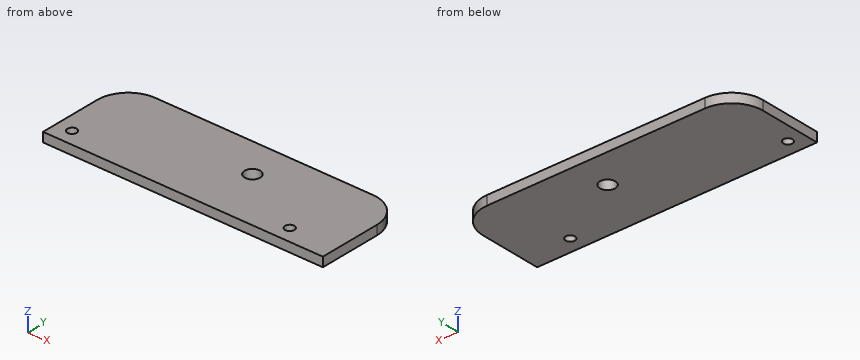
from build123d import *

# Parameters (mm, degrees)
SKETCH_1_W          = 90
SKETCH_1_H          = 30
EXTRUDE_1_DEPTH     = 3
SKETCH_3_R          = 2.5
CUT_EXTRUDE_2_DEPTH = 10
SKETCH_4_R          = 1.5
CUT_EXTRUDE_3_DEPTH = 10
FILLET_1_R          = 10


with BuildPart() as part:
    # 草图1 → 凸台-拉伸1 (new body)
    with BuildSketch(Plane.XY):
        Rectangle(SKETCH_1_W, SKETCH_1_H)
    extrude(amount=EXTRUDE_1_DEPTH)

    # 草图3 → 切除-拉伸2 (cut)
    with BuildSketch(Plane.XY.offset(3)):
        with Locations((6.49227102, 3.236967106)):
            Circle(SKETCH_3_R)
    extrude(amount=-CUT_EXTRUDE_2_DEPTH, mode=Mode.SUBTRACT)

    # 草图4 → 切除-拉伸3 (cut)
    with BuildSketch(Plane.XY.offset(3)):
        with Locations((-40, -10)):
            Circle(SKETCH_4_R)
        with Locations((30, -10)):
            Circle(SKETCH_4_R)
    extrude(amount=-CUT_EXTRUDE_3_DEPTH, mode=Mode.SUBTRACT)

    # 圆角1
    fillet_1_edges = [part.edges().sort_by_distance(p)[0] for p in [
        (-45, 15, 1.5),
        (45, 15, 1.5),
    ]]
    fillet(fillet_1_edges, radius=FILLET_1_R)


solid = part.part
Can you work these out from the model? Positions are in its coordinate system, mm. Coordinates: 2 decimals unless noted, no trailing zeros. Write each loop counter-clockwise with the first axis right and the second up, starting at its lowest first coordinate (ties: lowest second). Pieces come first, ordered by that corner, then holes. Notation, with made-up numbers: (64, -12.75) - (94, -12.75) arc R15 cw to (94, 15.25) - close; hole circle Ø1 at (50.25, 81.5). An arc over 180 degrees is marked (long way). Return JSON: item names as keys, results as strings. Group by question number.
Item 1: If we section it at B-B (x = 30): Write out the boundary of the cut face in (y, z), then the cut area to 3 significant figures.
Item 2: If we section it at D-D (x = 5.5): Write out the boundary of the cut face in (y, z).
Item 3: If we section it at A-A (y = -10): Write out the boundary of the cut face in (x, z), then the cut area to 3 significant figures.
Item 4: If we section it at C-C (z = 1.3): Write out the boundary of the cut face in (x, y).
Item 5: Please list where these lines run through material, in increasing order: probe 1 along Y at (x, z) = (30, 1.15); probe 2 along X at (y, z) = (2, 0.65); probe 3 along X at (y, z) = (2.5, 0.2).
Return value:
{
 "1": {"outline": "(-15, 0) - (-11.5, 0) - (-11.5, 3) - (-15, 3) - close; (-8.5, 0) - (15, 0) - (15, 3) - (-8.5, 3) - close", "area": "81.0 mm^2"},
 "2": {"outline": "(-15, 0) - (0.94, 0) - (0.94, 3) - (-15, 3) - close; (5.53, 0) - (15, 0) - (15, 3) - (5.53, 3) - close"},
 "3": {"outline": "(-45, 0) - (-41.5, 0) - (-41.5, 3) - (-45, 3) - close; (-38.5, 0) - (28.5, 0) - (28.5, 3) - (-38.5, 3) - close; (31.5, 0) - (45, 0) - (45, 3) - (31.5, 3) - close", "area": "252 mm^2"},
 "4": {"outline": "(-45, -15) - (45, -15) - (45, 5) arc R10 ccw to (35, 15) - (-35, 15) arc R10 ccw to (-45, 5) - close; hole circle Ø3 at (-40, -10); hole circle Ø5 at (6.49, 3.24); hole circle Ø3 at (30, -10)"},
 "5": {"probe 1": "y = -15 to -11.5, -8.5 to 15", "probe 2": "x = -45 to 4.32, 8.66 to 45", "probe 3": "x = -45 to 4.1, 8.88 to 45"}
}
